from build123d import *

# Parameters (mm, degrees)
BOSS_EXTRUDE1_DEPTH = 150
FILLET1_R           = 1


with BuildPart() as part:
    # Sketch1 → Boss-Extrude1 (new body)
    with BuildSketch(Plane(origin=(0, 0, 0), x_dir=(1, 0, 0), z_dir=(0, 1, 0))):
        with BuildLine():
            Line((-42, 0), (-40, 0))
            ThreePointArc((-40, 0), (-18.181666667, -21.818333333), (3.636666667, 0))
            Line((3.636666667, 0), (5.636666667, 0))
            ThreePointArc((5.636666667, 0), (-18.181666667, -23.818333333), (-42, 0))
        make_face()
    extrude(amount=BOSS_EXTRUDE1_DEPTH)

    # Fillet1
    fillet1_edges = [part.edges().sort_by_distance(p)[0] for p in [
        (5.636666667, 75, 0),
        (3.636666667, 75, 0),
        (-40, 75, 0),
        (-42, 75, 0),
    ]]
    fillet(fillet1_edges, radius=FILLET1_R - 0.0001)  # a hair under: the kernel refuses the full size


solid = part.part
The listing builds one solid part. Answer for the finished solid, in the listing's coordinates (mm). Give positions to 0.01 mm unless a question says otherwise; leave off trailing zeros. Order: outer loops, then holes, each group sorted by start corner. A loop starts at its lowest first (then second) coordinate and runs counter-clockwise, first axis right, second up. Notation, with made-up numbers: (7.5, 9.25) - (17.5, 9.25) arc R9 ccw to (17.5, 15.25) - close; hole circle Ø9 at (15, -35). An arc over 180 degrees is marked (long way). One line per item, written item: value. Start each with the question number.
1) A cutting plane is placed at C-C on z = 16.75. Give the vertices of the cut face in (x, y), then the cut area to 3 significant figures.
2) Find the intervals of material crossed by L1, parallel to Z at x = -18, y = 42.5; L2, parallel to X at y = 66, z = 4.5; L3, parallel to X at y = 24, z = 19.5, in increasing order.
3) The mould has two halves that part along X. Classify faces 1 (the face through (-18.648, 73.95, 21.813)), 2 (the face through (-15, 150, 22)), 3 (the face through (-17.673, 73.95, 23.813)): released by +X, released by -X, zero draft, split by the parting line, or undercut.
4) A cutting plane is placed at D-D on x = -17. Give the vertices of the cut face in (y, z).
5) Given pin 1 Ø2 at (x, y) = (-3.5, 126.5) entering from +Z; pin 2 Ø2 at (y, z) = (116.5, 16) entering from +X; pin 3 Ø6 at (x, y) = (-16, 120) entering from -Z, each flat-ended and moving along its own axis, determine where each tip first touches the part or whether it passes through.
6) A cutting plane is placed at A-A on z = 7.75. Give the vertices of the cut face in (x, y), then the cut area to 3 significant figures.
Answer sheet:
1. outline: (-35.12, 0) - (-32.16, 0) - (-32.16, 150) - (-35.12, 150) - close; (-4.2, 0) - (-1.25, 0) - (-1.25, 150) - (-4.2, 150) - close
1. area: 886 mm2
2. L1: z = 21.82 to 23.82
2. L2: x = -41.57 to -39.53, 3.17 to 5.21
2. L3: x = -31.86 to -27.97, -8.39 to -4.5
3. face 1: undercut
3. face 2: zero draft
3. face 3: split by the parting line
4. outline: (0, 21.79) - (150, 21.79) - (150, 23.79) - (0, 23.79) - close
5. pin 1: stops at z = 19.5
5. pin 2: stops at x = 0.32
5. pin 3: stops at z = 21.19
6. outline: (-40.7, 0) - (-38.58, 0) - (-38.58, 150) - (-40.7, 150) - close; (2.21, 0) - (4.34, 0) - (4.34, 150) - (2.21, 150) - close
6. area: 638 mm2
